```python
from build123d import *

# Parameters (mm, degrees)
SKETCH_1_R          = 6
EXTRUDE_1_DEPTH     = 8
EXTRUDE_1_2_DEPTH   = 8
EXTRUDE_1_3_DEPTH   = 8
SKETCH_3_R          = 2.5
CUT_EXTRUDE_1_DEPTH = 128.141653285
SKETCH_4_R          = 2
CUT_EXTRUDE_2_DEPTH = 128.141653285
SKETCH_5_R          = 4
CUT_EXTRUDE_3_DEPTH = 4.5
FILLET_1_R          = 10


with BuildPart() as part:
    # 草图1 → Extrude 1 (new body)
    with BuildSketch(Plane.XY):
        Circle(SKETCH_1_R)
    extrude(amount=EXTRUDE_1_DEPTH)



with BuildPart() as body_2:
    # 草图1 → Extrude 1 2 (new body)
    with BuildSketch(Plane.XY):
        with Locations((0, 120)):
            Circle(SKETCH_1_R)
    extrude(amount=EXTRUDE_1_2_DEPTH)


with BuildPart() as part_1:
    add(part.part)

    add(body_2.part)  # Extrude 1 3 merges body 2
    # 草图2 → Extrude 1 3 (add)
    with BuildSketch(Plane.XY):
        Polygon((-4.330127019, 117.5), (5, 101.339745962), (5, 18.660254038), (-4.330127019, 2.5), (4.330127019, -2.5), (15, 15.980762114), (15, 104.019237886), (4.330127019, 122.5), align=None)
    extrude(amount=EXTRUDE_1_3_DEPTH)

    # 草图3 → 切除-拉伸1 (cut, through all)
    with BuildSketch(Plane.XY.offset(8)):
        with Locations((0, 120)):
            Circle(SKETCH_3_R)
    extrude(amount=-CUT_EXTRUDE_1_DEPTH, mode=Mode.SUBTRACT)

    # 草图4 → 切除-拉伸2 (cut, through all)
    with BuildSketch(Plane.XY.offset(8)):
        Circle(SKETCH_4_R)
    extrude(amount=-CUT_EXTRUDE_2_DEPTH, mode=Mode.SUBTRACT)

    # 草图5 → 切除-拉伸3 (cut)
    with BuildSketch(Plane.XY.offset(8)):
        Circle(SKETCH_5_R)
    extrude(amount=-CUT_EXTRUDE_3_DEPTH, mode=Mode.SUBTRACT)

    # 圆角1
    fillet_1_edges = [part_1.edges().sort_by_distance(p)[0] for p in [
        (5, 18.660254038, 4),
        (15, 15.980762114, 4),
        (15, 104.019237886, 4),
        (5, 101.339745962, 4),
    ]]
    fillet(fillet_1_edges, radius=FILLET_1_R)


solid = part_1.part
```
Geometry check sheet. Reference: the model listing, model coordinates, mm. A direction names the side the tool comes from. Give positions to 0.01 mm unless a question says otherwise; leave off trailing zeros. Write each loop counter-clockwise with the first axis right and the second up, starting at its lowest first coordinate (ties: lowest second). Pieces come first, ordered by that corner, then holes.
1) Material ranges on L1, parallel to X at y = 57.5, z = 2.5; L2, parallel to Y at x = 0, z = 1.75; L3, parallel to Y at x = 0, z = 5, recorded low to high.
2) Gauge pin test, flat ends, axial feed: pin 1 (3 mm diameter, centred on y = 94, z = 7, fed in from -X); pin 2 (10.5 mm diameter, centred on x = 0, y = 0, fed in from +Z); pin 3 (2.5 mm diameter, centred on x = -1.5, y = -0.5, fed in from +Z); pin 4 (1.5 mm diameter, centred on x = 4, z = 6.5, fed in from -Y). Record the tip position at first contact, or that the pin passes through.
3) Access from +Z, -Z, +X, -X, +Y, -Y to the whole of each face (thin tool, end or side, straight path). Record for faces 1 (the cylindrical face through (4.65, 101.28, 4.06)), 2 (the cylindrical face through (-0.867, -3.905, 5.781)), 3 (the cylindrical face through (14.67, 16.11, 4.06)).
4) Release check for a two-part mould opening along Y. For faces 4 (the flat face through (0.45, 109.22, 3.94)), 5 (the flat face through (9.88, 112.89, 3.94)), 6 (the flat face through (9.77, 6.92, 3.94)) record: pulls with the +Y half, pulls with the -Y half, needs draft (parallel to the pull), parting line crosses it, or undercut.
5) Section check A-A, the plane x = 0. Record the boundary of the cut face in (y, z), and give its area (3 significant figures).
6) Section check B-B, the plane z = 1.5. Record the boundary of the cut face in (x, y), and give its area (3 significant figures).
7) Section check D-D, the plane y = 105. Record the boundary of the cut face in (x, z).
8) Section check C-C, the plane y = 26.5. Record the boundary of the cut face in (x, z), and give its area (3 significant figures).
Computed:
1. L1: x = 5 to 15
1. L2: y = -6 to -2, 2 to 10, 110 to 117.5, 122.5 to 126
1. L3: y = -6 to -4, 4 to 10, 110 to 117.5, 122.5 to 126
2. pin 1: stops at x = 5
2. pin 2: stops at z = 8
2. pin 3: stops at z = 3.5
2. pin 4: stops at y = -5.04
3. face 1: +Z, -Z, -X
3. face 2: +Z
3. face 3: +Z, -Z, +X, -Y
4. face 4: undercut
4. face 5: pulls with the +Y half
4. face 6: pulls with the -Y half
5. outline: (-6, 0) - (-2, 0) - (-2, 3.5) - (-4, 3.5) - (-4, 8) - (-6, 8) - close; (2, 0) - (10, 0) - (10, 8) - (4, 8) - (4, 3.5) - (2, 3.5) - close; (110, 0) - (117.5, 0) - (117.5, 8) - (110, 8) - close; (122.5, 0) - (126, 0) - (126, 8) - (122.5, 8) - close
5. area: 166 mm2
6. outline: (-2.67, 5.37) arc R6 ccw (long way) to (5.99, 0.37) - (13.66, 13.66) arc R10 ccw to (15, 18.66) - (15, 101.34) arc R10 ccw to (13.66, 106.34) - (5.99, 119.63) arc R6 ccw (long way) to (-2.67, 114.63) - (3.66, 103.66) arc R10 cw to (5, 98.66) - (5, 21.34) arc R10 cw to (3.66, 16.34) - close; hole circle Ø5 at (0, 120); hole circle Ø4 at (0, 0)
6. area: 1,340 mm2
7. outline: (2.89, 0) - (14.31, 0) - (14.31, 8) - (2.89, 8) - close
8. outline: (5, 0) - (15, 0) - (15, 8) - (5, 8) - close
8. area: 80.0 mm2
